Autodesk Inventor part; units mm, degrees
ref_plane "YZ Plane" through (0, 0, 0) normal (1, 0, 0) x (0, 1, 0)
ref_plane "XZ Plane" through (0, 0, 0) normal (0, 1, 0) x (-1, 0, 0)
ref_plane "XY Plane" through (0, 0, 0) normal (0, 0, 1) x (1, 0, 0)
sketch "Sketch1" plane through (0, 0, 0) normal (1, 0, 0) x (0, 1, 0)
  line L0 (0, 5.2) -> (6.6, 5.2)
  line L1 (6.6, 5.2) -> (6.6, 4.7)
  line L2 (2.5, 0.6) -> (2.5, -0.9618)
  line L3 (2.5, -0.9618) -> (0, -0.9618)
  line L4 (0, -0.9618) -> (0, 0.9)
  line L5 (0, 0.9) -> (1.5, 0.9)
  line L6 (1.5, 0.9) -> (1.5, 4.5)
  line L7 (1.5, 4.5) -> (0, 4.5)
  line L8 (0, 4.5) -> (0, 5.2)
  line L9 (6.6, 4.7) -> (2.5, 0.6)
  point P0 (0, 0)
  point P1 (1.5, 2.7)
  point P2 (0, 0)
  dimension "d0" = 3.6
  dimension "d1" = 1.5
  dimension "d2" = 6.6
  dimension "d3" = 45
  dimension "d4" = 5.2
  dimension "d6" = 2.7
  dimension "d7" = 0
  dimension "d8" = 1
  dimension "d9" = 0.5
extrude "Extrusion1" add sketch "Sketch1" along normal mid plane 4.5
sketch "Sketch2" plane through (-2.25, 0, 5.2) normal (0, 0, 1) x (1, 0, 0)
  line L0 (2.25, 0) -> (2.25, 10.2) construction
  circle A0 centre (2.25, 5.1) radius 1.5
  line L1 (4.5, 6.6) -> (0, 6.6)
  dimension "d12" = 3
extrude "Extrusion2" add sketch "Sketch2" along normal blind 3.8
fillet "Fillet1" radius 1.5 1 edges at (-1.5, 5.1, 9)
sketch "Sketch3" plane through (-2.25, 0, -0.9618) normal (0, -1, 0) x (1, 0, 0)
  circle A0 centre (1, 0.9618) radius 0.65
  circle A1 centre (3.5, 0.9618) radius 0.65
  line L0 (0, 6.1618) -> (4.5, 6.1618)
  point P0 (2.25, 0.9618)
  dimension "d16" = 1.3
  dimension "d17" = 1.3
  dimension "d18" = 5.2
  dimension "d19" = 1.25
  dimension "d20" = 1.25
  dimension "d21" = 5.2
extrude "Extrusion3" add sketch "Sketch3" along normal blind 1.6
properties part number "SLP3"
Input: part model. Units: mm. Frame: model coordinates. A direction names the side the tool comes from. Give positions to 0.01 mm unless a question says otherwise; leave off trailing zeros. Order: outer loops, then holes, each group sorted by start corner. A loop starts at its lowest first (then second) coordinate and runs counter-clockwise, first axis right, second up.
1. Pin query (flat end, axial travel): pin 1 Ø1.8 at (x, z) = (0, 3) entering from -Y. Return the tip coordinate at first contact, or that it passes through.
Computed:
pin 1: stops at y = 1.5
2. Cut plane C-C (y = 5.1). Return loops of the section in (x, z).
Computed:
outline: (-2.25, 3.2) - (2.25, 3.2) - (2.25, 5.2) - (1.5, 5.2) - (1.5, 7.5) arc R1.5 ccw to (-1.5, 7.5) - (-1.5, 5.2) - (-2.25, 5.2) - close
3. Cut plane B-B (z = 0). Return loops of the section in (x, y), and give its area (3 significant figures).
Computed:
outline: (-2.25, 0) - (-1.9, 0) - (-1.9, -1.6) - (-0.6, -1.6) - (-0.6, 0) - (0.6, 0) - (0.6, -1.6) - (1.9, -1.6) - (1.9, 0) - (2.25, 0) - (2.25, 2.5) - (-2.25, 2.5) - close
area: 15.4 mm2
4. Line query: probe 1 along Y at (x, z) = (0.4, 0); probe 2 along Z at (x, y) = (-1.1, 1.75); probe 3 along Z at (x, y) = (1.2, -0.5). Output: solid intervals per line, ascending.
Computed:
probe 1: y = 0 to 2.5
probe 2: z = -0.96 to 5.2
probe 3: z = -0.65 to 0.65
5. Cut plane D-D (x = 1). Return loops of the section in (y, z), and give its area (3 significant figures).
Computed:
outline: (-1.6, -0.6) - (0, -0.6) - (0, -0.96) - (2.5, -0.96) - (2.5, 0.6) - (6.6, 4.7) - (6.6, 5.2) - (6.22, 5.2) - (6.22, 7.5) arc R1.12 ccw to (3.98, 7.5) - (3.98, 5.2) - (0, 5.2) - (0, 4.5) - (1.5, 4.5) - (1.5, 0.9) - (0, 0.9) - (0, 0.6) - (-1.6, 0.6) - close
area: 29.5 mm2
6. Set-up query: faces 5 (the face through (0, 2.5, 0)), 6 (the face through (0, 1.5, 3)), 7 (the face through (-0.63, -0.79, -0.2)). Return all of +Z, -Z, +X, -X, +Y, -Y with unobstructed straight access to the full face (end or side cutting, diameter ignored); none if empty.
Computed:
face 5: -Z, +X, -X, +Y
face 6: +X, -X, -Y
face 7: -Y
7. Cut plane A-A (y = 0.5). Return loops of the section in (x, z).
Computed:
outline: (-2.25, -0.96) - (2.25, -0.96) - (2.25, 0.9) - (-2.25, 0.9) - close; (-2.25, 4.5) - (2.25, 4.5) - (2.25, 5.2) - (-2.25, 5.2) - close
8. Draft query along X for faces 1 (the face through (0.6, -0.8, 0)), 2 (the face through (2.25, 3, 3)), 3 (the face through (0, 4.6, 2.7)), 4 (the face through (-0.325, 6.564, 6.334)). Return one class per face: released by +X, released by -X, zero draft, split by the parting line, or undercut.
Computed:
face 1: undercut
face 2: released by +X
face 3: zero draft
face 4: split by the parting line
